Part model, mm, in its own coordinate system. Face numbers are marked on the shaded views. A direction names the side the tool comes from. Give positions to 0.01 mm unless a question says otherwise; leave off trailing zeros. Loops run counter-clockwise (first coordinate to the right, second up) from the corner with the lowest first, then second, coordinate; pieces in that order, holes last. Notation, with made-up numbers: M -21.75,46 L 29.25,46 A4 cw 29.25,53 Z; hole C 87.25,19.5 d9. An arc over 180 degrees is marked long. Put each result on its own line as item: value. Start each with the question number.
```python
from build123d import *

# Parameters (mm, degrees)
SKETCH_1_R      = 19
EXTRUDE_1_DEPTH = 12
SKETCH_2_R      = 10
EXTRUDE_2_DEPTH = 6
SKETCH_3_R      = 5
EXTRUDE_3_DEPTH = 20


with BuildPart() as part:
    # 草图1 → 凸台-拉伸1 (new body)
    with BuildSketch(Plane(origin=(0, 0, 0), x_dir=(1, 0, 0), z_dir=(0, 1, 0))):
        Circle(SKETCH_1_R)
    extrude(amount=EXTRUDE_1_DEPTH)

    # 草图2 → 凸台-拉伸2 (add)
    with BuildSketch(Plane(origin=(0, 12, 0), x_dir=(1, 0, 0), z_dir=(0, 1, 0))):
        Circle(SKETCH_2_R)
    extrude(amount=EXTRUDE_2_DEPTH)

    # 草图3 → 凸台-拉伸3 (add)
    with BuildSketch(Plane(origin=(0, 18, 0), x_dir=(1, 0, 0), z_dir=(0, 1, 0))):
        Circle(SKETCH_3_R)
    extrude(amount=EXTRUDE_3_DEPTH)


solid = part.part
```
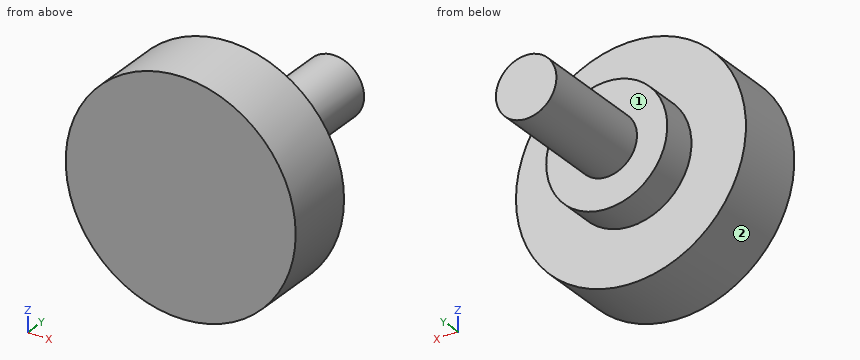
1) Band-saw the part on A-A on z = 0. Give the cut face in (x, y), then the cut area to 3 significant figures.
2) Which spindle directions (+Z, -Z, +X, -X, +Y, -Y) get a long thin tool onto all of the face, cutting with end or side? Do the marked faces 1 and 2. Say none if no direction does.
3) Band-saw the part on D-D on x = -6.5. Give the cut face in (y, z).
4) Band-saw the part on B-B on x = 0. Give the cut face in (y, z), then the cut area to 3 significant figures.
5) Band-saw the part on C-C on y = 4. Give the cut face in (x, z), then the cut area to 3 significant figures.
6) Wall check: L1, parallel to Y at x = -2, z = -15.5; L2, parallel to Y at x = 5, z = 6; L3, parallel to X at y = 12.5, z = -3. Give the ranges that are in metal, low to high.
7) Pin check, flat tips, straight feed: pin 1 Ø1.5 at (x, z) = (12.5, -14.5) entering from -Y; pin 2 Ø8 at (y, z) = (26, -8.5) entering from +X; pin 3 Ø3 at (x, y) = (4, 32.5) entering from -Z; pin 4 Ø5 at (y, z) = (4.5, 6) entering from -X. Stop position of each tip, or through.
Evaluation:
1. outline: M -19,0 L 19,0 L 19,12 L 10,12 L 10,18 L 5,18 L 5,38 L -5,38 L -5,18 L -10,18 L -10,12 L -19,12 Z
1. area: 776 mm2
2. face 1: +Y
2. face 2: +Y, -Y
3. outline: M 0,-17.85 L 12,-17.85 L 12,-7.6 L 18,-7.6 L 18,7.6 L 12,7.6 L 12,17.85 L 0,17.85 Z
4. outline: M 0,-19 L 12,-19 L 12,-10 L 18,-10 L 18,-5 L 38,-5 L 38,5 L 18,5 L 18,10 L 12,10 L 12,19 L 0,19 Z
4. area: 776 mm2
5. outline: C 0,0 d38
5. area: 1,130 mm2
6. L1: 0 to 12
6. L2: 0 to 18
6. L3: -9.54 to 9.54
7. pin 1: y = 0
7. pin 2: x = 2.18
7. pin 3: z = -4.33
7. pin 4: x = -18.67
